Verification items for this drawing (mm, ordinates from the low corner). A direction names the side the tool comes from. Coordinates: 2 decimals unless noted, no trailing zeros. Order: outer loops, then holes, each group sorted by start corner. A loop starts at its lowest first (then second) coordinate and runs counter-clockwise, first axis right, second up.
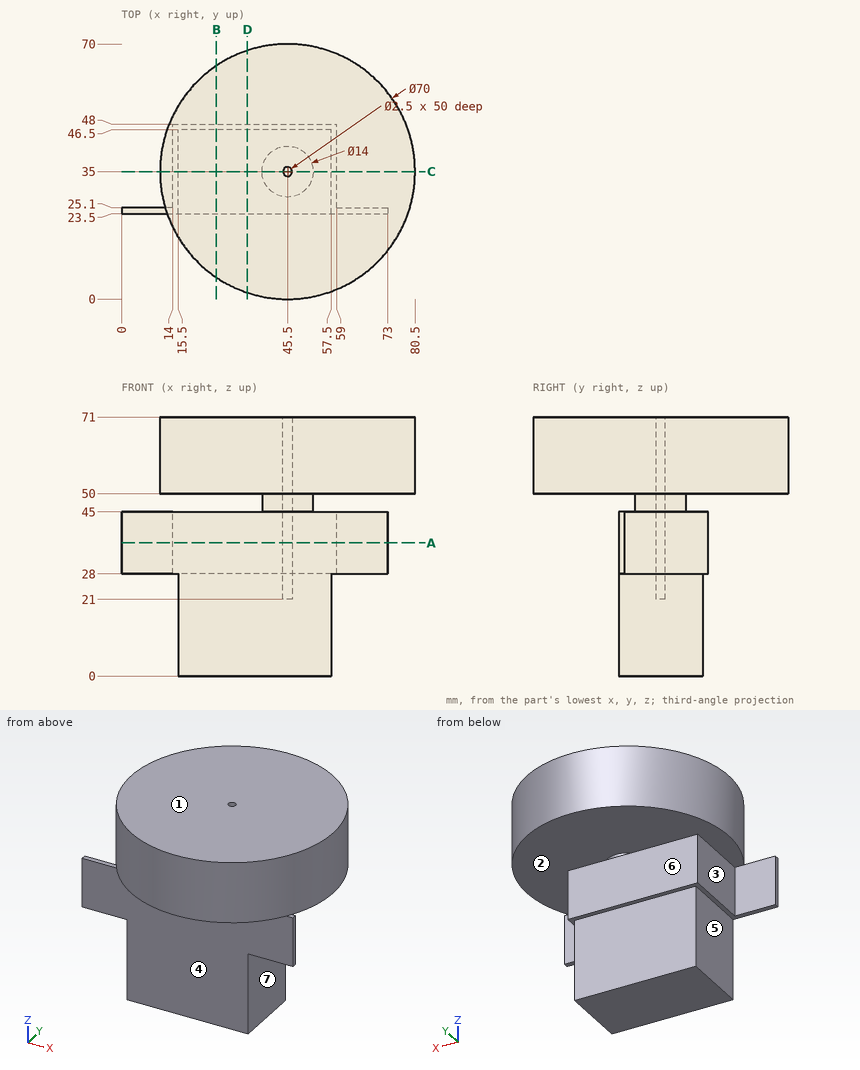
(1) Thickness scan on probe 1 along Y at (x, z) = (45.5, 33); probe 2 along Y at (x, z) = (45.5, 53.5); probe 3 along X at (y, z) = (31, 22.5). Record the ranges inside material, lowest first.
Filled in:
probe 1: y = 23.5 to 33.75, 36.25 to 48
probe 2: y = 0 to 33.75, 36.25 to 70
probe 3: x = 15.5 to 57.5
(2) Go/stop test with flat-tipped pins: P1, Ø15.5, axis at x = 4.5, z = 38.5, coming from the +Y side; P2, Ø3, axis at x = 10, y = 25, coming from the -Z side; P3, Ø8.5, axis at x = 26.5, z = 33, coming from the +Y side. Record where each tip stops, or that it passes through.
Filled in:
P1: stops at y = 25.1
P2: stops at z = 28
P3: stops at y = 48
(3) Release check for a two-part mould opening along Z. For the marked faces 1, 2 and 3 record: +Z half, -Z half, draft (parallel to the pull), parting line (faces both ways), or undercut.
Filled in:
face 1: +Z half
face 2: undercut
face 3: draft
(4) Cross-section at D-D (x = 34.5). Enter the section's corners in (y, z).
Filled in:
outline: (1.77, 50) - (68.23, 50) - (68.23, 71) - (1.77, 71) - close; (23.5, 0) - (46.5, 0) - (46.5, 28) - (48, 28) - (48, 45) - (23.5, 45) - close
(5) Cross-section at A-A (z = 36.5). Enter the section's corners in (x, y).
Filled in:
outline: (0, 23.5) - (73, 23.5) - (73, 25.1) - (59, 25.1) - (59, 48) - (14, 48) - (14, 25.1) - (0, 25.1) - close; hole circle Ø2.5 at (45.5, 35)
(6) Tool access check on the marked faces 4, 5, 6 and 7. Record the directions out of +Z, -Z, +X, -X, +Y, -Y that give a thin tool (end or side, any length) a straight path to the whole face; none if there is none.
Filled in:
face 4: -Z, +X, -X, -Y
face 5: -Z, -X, +Y, -Y
face 6: -Z, +X, -X, +Y
face 7: -Z, +X, +Y, -Y
(7) Cross-section at C-C (y = 35). Enter the section's corners in (x, z).
Filled in:
outline: (10.5, 50) - (38.5, 50) - (38.5, 45) - (14, 45) - (14, 28) - (15.5, 28) - (15.5, 0) - (57.5, 0) - (57.5, 28) - (59, 28) - (59, 45) - (52.5, 45) - (52.5, 50) - (80.5, 50) - (80.5, 71) - (46.75, 71) - (46.75, 21) - (44.25, 21) - (44.25, 71) - (10.5, 71) - close
(8) Cross-section at B-B (x = 26). Enter the section's corners in (y, z), and give its area (3 significant figures).
Filled in:
outline: (5.94, 50) - (64.06, 50) - (64.06, 71) - (5.94, 71) - close; (23.5, 0) - (46.5, 0) - (46.5, 28) - (48, 28) - (48, 45) - (23.5, 45) - close
area: 2,280 mm2
